from build123d import *

# Parameters (mm, degrees)
SKETCH1_R                = 1.75
BOSS_EXTRUDE1_DEPTH      = 1.5
BOSS_EXTRUDE2_DEPTH      = 72
BOSS_EXTRUDE3_DEPTH      = 1.5
BOSS_EXTRUDE3_DEPTH_BACK = 1.5
BOSS_EXTRUDE4_DEPTH      = 2
SKETCH5_R                = 1.75
CUT_EXTRUDE1_DEPTH       = 2
CUT_EXTRUDE2_DEPTH       = 148.332054879
CUT_EXTRUDE2_DEPTH_BACK  = 148.332054879
SKETCH6_W                = 72
SKETCH6_H                = 11.553195909
FILLET1_R                = 2
SKETCH8_W                = 35
SKETCH8_H                = 19.946804091
CUT_EXTRUDE3_DEPTH       = 22.4262221


with BuildPart() as part:
    # Sketch1 → Boss-Extrude1 (new body)
    with BuildSketch(Plane.XY):
        with BuildLine():
            Line((-31.5, -134.5), (31.5, -134.5))
            Line((31.5, -134.5), (36, -134.5))
            Line((36, -134.5), (36, -132.049019419))
            ThreePointArc((36, -132.049019419), (37.374296294, -129.5), (36, -126.950980581))
            Line((36, -126.950980581), (36, -6.049019419))
            ThreePointArc((36, -6.049019419), (37.33874188, -3.5), (36, -0.950980581))
            Line((36, -0.950980581), (36, 0))
            Line((36, 0), (-36, 0))
            Line((-36, 0), (-36, -0.950980581))
            ThreePointArc((-36, -0.950980581), (-37.339851511, -3.504206195), (-35.994020506, -6.054285021))
            Line((-35.994020506, -6.054285021), (-36, -126.950980581))
            ThreePointArc((-36, -126.950980581), (-37.376731289, -129.5), (-36, -132.049019419))
            Line((-36, -132.049019419), (-36, -134.5))
            Line((-36, -134.5), (-31.5, -134.5))
        make_face()
        with Locations((-34.328609587, -129.5)):
            Circle(SKETCH1_R, mode=Mode.SUBTRACT)
        with Locations((34.323211043, -129.5)):
            Circle(SKETCH1_R, mode=Mode.SUBTRACT)
        with Locations((34.242652207, -3.5)):
            Circle(SKETCH1_R, mode=Mode.SUBTRACT)
        with Locations((-34.244120111, -3.500578956)):
            Circle(SKETCH1_R, mode=Mode.SUBTRACT)
    extrude(amount=BOSS_EXTRUDE1_DEPTH)

    # Sketch2 → Boss-Extrude2 (add)
    with BuildSketch(Plane.ZY.offset(36)):
        Polygon((1.5, -134.5), (1.5, -136.7), (-40, -136.7), (-40, -134.7), (0, -134.7), (0, -134.5), (0, -132.049019419), (1.5, -132.049019419), align=None)
    extrude(amount=-BOSS_EXTRUDE2_DEPTH)

    # Sketch3 → Boss-Extrude3 (add, two sides: drawn at the far end of the back side and taken through both)
    with BuildSketch(Plane(origin=(0, 0, 0), x_dir=(0, 0, -1), z_dir=(1, 0, 0)).offset(-BOSS_EXTRUDE3_DEPTH_BACK)):
        Polygon((0, -119.7), (15, -134.7), (0, -134.7), align=None)
    extrude(amount=BOSS_EXTRUDE3_DEPTH + BOSS_EXTRUDE3_DEPTH_BACK)

    # Sketch4 → Boss-Extrude4 (add)
    with BuildSketch(Plane.XZ.offset(136.7)):
        with BuildLine():
            Line((-36, -17.152805247), (-36, -22.963011674))
            ThreePointArc((-36, -22.963011674), (-37.650416645, -20.05790846), (-36, -17.152805247))
        make_face()
        with BuildLine():
            Line((36, -17.152805247), (36, -22.963011674))
            ThreePointArc((36, -22.963011674), (37.68082264, -20.05790846), (36, -17.152805247))
        make_face()
    extrude(amount=-BOSS_EXTRUDE4_DEPTH)

    # Sketch5 → Cut-Extrude1 (cut)
    with BuildSketch(Plane.XZ.offset(136.7)):
        with Locations(Location((-34.253947115, -19.946804091, 0), (0, 0, 270))):
            Circle(SKETCH5_R)
        with Locations(Location((34.288977705, -19.889159472, 0), (0, 0, 270))):
            Circle(SKETCH5_R)
    extrude(amount=-CUT_EXTRUDE1_DEPTH, mode=Mode.SUBTRACT)

    # Sketch6 → Cut-Extrude2 (cut, two sides: drawn at the far end of the back side and taken through both)
    with BuildSketch(Plane.XZ.offset(136.7).offset(-CUT_EXTRUDE2_DEPTH_BACK)):
        with Locations((0, -34.223402046)):
            Rectangle(SKETCH6_W, SKETCH6_H)
    extrude(amount=CUT_EXTRUDE2_DEPTH + CUT_EXTRUDE2_DEPTH_BACK, mode=Mode.SUBTRACT)

    # Fillet1
    fillet1_edges = [part.edges().sort_by_distance(p)[0] for p in [
        (36, -135.7, -28.446804091),
        (-36, -135.7, -28.446804091),
    ]]
    fillet(fillet1_edges, radius=FILLET1_R)

    # Sketch8 → Cut-Extrude3 (cut)
    with BuildSketch(Plane.XZ.offset(136.7)):
        with Locations((-13.5, -15.473402046)):
            Rectangle(SKETCH8_W, SKETCH8_H)
    extrude(amount=-CUT_EXTRUDE3_DEPTH, mode=Mode.SUBTRACT)


solid = part.part
CAD build for the part. Positions are in the model's coordinates, mm. A direction names the side the tool comes from. Coordinates: 2 decimals unless noted, no trailing zeros. Loops run counter-clockwise (first coordinate to the right, second up) from the corner with the lowest first, then second, coordinate; pieces in that order, holes last. Notation, with made-up numbers: (-28.5, 49) - (-14.5, 49) arc R14 cw to (-14.5, 69) - close; hole circle Ø6 at (-34, 42). An arc over 180 degrees is marked (long way). Write item = value, one per line. Start each with the question number.
Q1. Drill centre lines: L1, parallel to X at y = -129.5, z = 0.5; L2, parallel to Z at x = 21, y = -65; L3, parallel to Y at x = 24, z = -8.75. Where is each one in solid material? Low to high.
Q2. Cut at A-A, the plane x = -27.5. List the corners of the cut face in (y, z).
Q3. Cut at B-B, the plane y = -129.5. List the corners of the cut face in (x, z), then the cut area to 3 significant figures.
Q4. Flat gauge pins, fed straight in: pin 1 Ø0.6 at (y, z) = (-135.5, -24.5) entering from +X; pin 2 Ø4 at (x, z) = (-34.25, -19.95) entering from +Y; pin 3 Ø0.8 at (y, z) = (-0.5, 1) entering from -X. Where does each tip first touch, or does it go through?
Q5. Cut at D-D, the plane z = -19.5. List the corners of the cut face in (x, y), then the cut area to 3 significant figures.
Q6. Cut at C-C, the plane z = -12. List the corners of the cut face in (x, y).
Q7. Pull direction Y, two halves, no side cores. Call faces 1 (the cylindrical face through (-33.52, -131.05, 0.74)), 2 (the flat face through (-1.5, -129, -3)), 3 (the flat face through (8, -136.7, -13)): pulls with the +Y half, pulls with the -Y half, needs draft (parallel to the pull), parting line crosses it, or undercut.
Q8. Which spindle directions (+Z, -Z, +X, -X, +Y, -Y) get a long thin tool onto all of the face, cutting with end or side? Do faces 4 (the flat face through (1.5, -129, -3)), 5 (the flat face through (-10, -135, -5.5)), 6 (the flat face through (8, -134.7, -14)), 7 (the flat face through (36, -135, -8)), 8 (the flat face through (-36, -135, -8)). Say none if no direction does.
Computed:
q1.L1 = -37.38 to -36.08, -32.58 to 32.57, 36.07 to 37.37
q1.L2 = 0 to 1.5
q1.L3 = -136.7 to -134.7
q2.outline = (-136.7, -28.45) - (-134.7, -28.45) - (-134.7, -25.45) - (-136.7, -25.45) - close; (-136.7, -5.5) - (-134.7, -5.5) - (-134.7, 0) - (0, 0) - (0, 1.5) - (-136.7, 1.5) - close
q3.outline = (-37.38, 0) - (-36.08, 0) - (-36.08, 1.5) - (-37.38, 1.5) - close; (-32.58, 0) - (-1.5, 0) - (-1.5, -5.5) - (1.5, -5.5) - (1.5, 0) - (32.57, 0) - (32.57, 1.5) - (-32.58, 1.5) - close; (36.07, 0) - (37.37, 0) - (37.37, 1.5) - (36.07, 1.5) - close
q3.area = 118 mm²
q4.pin_1 = 36
q4.pin_2 = -134.7
q4.pin_3 = -36
q5.outline = (-37.6, -136.7) - (-35.95, -136.7) - (-35.95, -134.7) - (-37.6, -134.7) - close; (-32.56, -136.7) - (-31, -136.7) - (-31, -134.7) - (-32.56, -134.7) - close; (4, -136.7) - (32.58, -136.7) - (32.58, -134.7) - (4, -134.7) - close; (36, -136.7) - (37.63, -136.7) - (37.63, -134.7) - (36, -134.7) - close
q5.area = 66.9 mm²
q6.outline = (-36, -136.7) - (-31, -136.7) - (-31, -134.7) - (-36, -134.7) - close; (4, -136.7) - (36, -136.7) - (36, -134.7) - (4, -134.7) - close
q7.face_1 = undercut
q7.face_2 = needs draft
q7.face_3 = pulls with the -Y half
q8.face_4 = -Z, +X, +Y
q8.face_5 = +Y, -Y
q8.face_6 = -Z, +Y
q8.face_7 = +Z, +X, -Y
q8.face_8 = +Z, -X, -Y
